from build123d import *

# Parameters (mm, degrees)
F0_R      = 25
F1_DEPTH  = 180
F2_R      = 20
F3_DEPTH  = 65
F4_W      = 10
F4_H      = 3.1937984634
F5_DEPTH  = 61.7
F7_D      = 24.16
F7_DEPTH  = 75
F7_TIP    = 7.2583962779
F8_W      = 10
F8_H      = 5.6645046324
F9_DEPTH  = 70
F11_R     = 2
F12_DEPTH = 25
F13_R     = 3.75
F14_DEPTH = 6


with BuildPart() as f1:
    # F0 (on Front) → F1 (new body)
    with BuildSketch(Plane.XZ):
        Circle(F0_R)
    extrude(amount=F1_DEPTH)

    # F2 (on face) → F3 (join)
    with BuildSketch(Plane.XZ.offset(180)):
        Circle(F2_R)
    extrude(amount=F3_DEPTH)

    # F4 (on face) → F5 (cut)
    with BuildSketch(Plane.XZ.offset(245)):
        with Locations((0, 20.9618159628)):
            Rectangle(F4_W, F4_H)
    extrude(amount=-F5_DEPTH, mode=Mode.SUBTRACT)

    # F7
    with Locations(Plane(origin=(0, 0, 0), x_dir=(-1, 0, 0), z_dir=(0, 1, 0))):
        with Locations((0, 0)):
            Hole(F7_D / 2, depth=F7_DEPTH)
            with Locations((0, 0, -(F7_DEPTH + F7_TIP / 2))):  # 118° drill point
                Cone(0, F7_D / 2, F7_TIP, mode=Mode.SUBTRACT)

    # F8 (on face) → F9 (cut)
    with BuildSketch(Plane(origin=(0, 0, 0), x_dir=(-1, 0, 0), z_dir=(0, 1, 0))):
        with Locations((0, 11.6677476838)):
            Rectangle(F8_W, F8_H)
    extrude(amount=-F9_DEPTH, mode=Mode.SUBTRACT)

    # F11 (on offset) → F12 (cut)
    with BuildSketch(Plane.XY.offset(25)):
        with Locations((0, -35)):
            Circle(F11_R)
    extrude(amount=-F12_DEPTH, mode=Mode.SUBTRACT)

    # F13 (on offset) → F14 (cut)
    with BuildSketch(Plane.XY.offset(25)):
        with Locations((0, -34.9959954619)):
            Circle(F13_R)
    extrude(amount=-F14_DEPTH, mode=Mode.SUBTRACT)


solid = f1.part
Can you work these out from the model? Positions are in its coordinate system, mm. A direction names the side the tool comes from. Give positions to 0.01 mm unless a question says otherwise; leave off trailing zeros. Write each loop counter-clockwise with the first axis right and the second up, starting at its lowest first coordinate (ties: lowest second). Pieces come first, ordered by that corner, then holes. Notation, with made-up numbers: (-18.75, 87.5) -> (14.25, 87.5) arc R16 ccw to (14.25, 95.5) -> close; hole circle Ø9 at (82, 35.5). An arc over 180 degrees is marked (long way). Answer as a JSON object with one key per item and string values. Group by question number.
Item 1: Please list where these lines run through material, in increasing order: line 1 (Y direction, x = 0, z = 16.95); line 2 (Z direction, x = 0, y = -22); line 3 (Z direction, x = 0, y = -75). Write a range as [from, to].
Item 2: For faces 1 (the face through (0, -215, 19.365)), 2 (the face through (0, -245, 0)), 3 (the face through (-4.336, -212.045, -19.524)), 4 (the face through (-2.619, -38.025, -11.793)), 5 (the face through (2, -37, 19)), which set-ups out of +Z, -Z, +X, -X, +Y, -Y let a thin tool reach every point of the face, with its end or its side?
Item 3: I'm going to push flat-ended pins straight in: P1, Ø2, axis at y = -37, z = -4.5, coming from the +X side; P2, Ø3, axis at y = -38.5, z = 12.5, coming from the -X side; P3, Ø8, axis at y = -143.5, z = 17, coming from the +X side. Where does each tip first touch, or does it pass through?
Item 4: Suppose I cut it at A-A (y = -205.5). Please give me the cut outline in (x, z), plus the area to 3 significant figures.
Item 5: We'd pull the mould along Y, two halves only. Please class faces 6 (the face through (1.73, -38.323, 22.042)), 7 (the face through (-2.2, -34.5, 14.5)), 8 (the face through (-6, 0, -11)), 9 (the face through (-11, -180, 17)): +Y half, -Y half, draft (parallel to the pull), parting line (faces both ways), or undercut.
Findings:
{
 "1": {"line 1": "y = [-245, -37], [-33, 0]", "line 2": "z = [-25, -12.08], [14.5, 25]", "line 3": "z = [-25, -12.08], [12.08, 25]"},
 "2": {"face 1": "+Z, +X, -X, -Y", "face 2": "+Z, -Z, +X, -X, -Y", "face 3": "-Y", "face 4": "+Y", "face 5": "+Z"},
 "3": {"P1": "stops at x = 24.75", "P2": "stops at x = -22.45", "P3": "stops at x = 21.35"},
 "4": {"outline": "(-5, 19.36) arc R20 ccw (long way) to (5, 19.36) -> close", "area": "1,250 mm²"},
 "5": {"face 6": "undercut", "face 7": "draft", "face 8": "+Y half", "face 9": "-Y half"}
}
